Here's how the part is built. I have some questions about the finished solid (model axes, mm). Round coordinates to 2 decimals unless told otherwise and drop trailing zeros. Write each loop counter-clockwise with the first axis right and the second up, starting at its lowest first coordinate (ties: lowest second). Pieces come first, ordered by that corner, then holes. Notation, with made-up numbers: (70, 32) - (90, 32) arc R18 ccw to (90, 55) - close; hole circle Ø9 at (29.5, 26.25). An arc over 180 degrees is marked (long way). Use one line per item in the form item = value. Start each with the question number.
1. I want a section at A-A, the plane x = 0. List the corners of the cut face in (y, z) for me, plus the area to 3 significant figures.
2. I want a section at C-C, the plane z = -65. List the corners of the cut face in (x, y) for me.
3. If I drill on line 1 along Z through (x, y) = (0, 2.25); line 2 along X through (y, z) = (1.25, -93.5); line 3 along X through (y, z) = (0, -108), over which ranges is the centre line in solid material (lowest first)?
4. Will these pins go through, and if not, where does the flat tip stop? pin 1 (4 mm diameter, centred on y = 1.5, z = -37, fed in from +X); pin 2 (3 mm diameter, centred on y = -2, z = -0.5, fed in from +X); pin 3 (3 mm diameter, centred on x = -1.5, y = 2.5, fed in from +Z); pin 4 (1.5 mm diameter, centred on x = -1.5, z = -55.5, fed in from -Y).
Autodesk Inventor part; units mm, degrees
ref_plane "FDT_KSAUFSATZ_XY" through (0, 0, 8.2) normal (0, 0, 1) x (-1, 0, 0)
ref_plane "FDT_KSAUFSATZ_YZ" through (0, 0, 8.2) normal (-1, 0, 0) x (0, -1, 0)
ref_plane "FDT_KSAUFSATZ_ZX" through (0, 0, 8.2) normal (0, -1, 0) x (0, 0, 1)
sketch "Sketch_2" plane through (0, 0, 0) normal (1, 0, 0) x (0, 1, 0)
  line L0 (0, -133.5) -> (0, 4)
  line L1 (0, 4) -> (2, 4)
  line L2 (2, 4) -> (2, -131.5)
  line L3 (2, -131.5) -> (4, -131.5)
  line L4 (4, -131.5) -> (4, -133.5)
  line L5 (4, -133.5) -> (0, -133.5)
  line L6 (0, -133.5) -> (0, 4)
revolve "Revolution1" add sketch "Sketch_2" angle 360 about axis through (0, 0, -133.5) along (0, 0, -1)
sketch "Sketch_6" plane through (0, 0, 0) normal (1, 0, 0) x (0, 1, 0)
  line L0 (0, 3) -> (0, 16)
  line L1 (0, 16) -> (1.5705, 16)
  line L2 (1.5705, 16) -> (2, 15.5705)
  line L3 (2, 15.5705) -> (2, 6.299)
  line L4 (2, 6.299) -> (1.6241, 5.2663)
  arc A0 (1.6241, 5.2663) -> (1.6, 5.1295) centre (2, 5.1295) ccw
  line L5 (1.6, 5.1295) -> (1.6, 4.4)
  arc A1 (1.6, 4.4) -> (2, 4) centre (2, 4.4) ccw
  line L6 (2, 4) -> (2, 3)
  line L7 (2, 3) -> (0, 3)
  line L8 (0, 3) -> (0, 16)
revolve "Revolution2" add sketch "Sketch_6" angle 360 about axis through (0, 0, 3) along (0, 0, -1)
thread "Thread1"
ref_plane "FDT_KSAUFSATZ_XY" through (0, 0, 8.2) normal (0, 0, 1) x (-1, 0, 0)
ref_plane "FDT_KSAUFSATZ_YZ" through (0, 0, 8.2) normal (-1, 0, 0) x (0, -1, 0)
ref_plane "FDT_KSAUFSATZ_ZX" through (0, 0, 8.2) normal (0, -1, 0) x (0, 0, 1)
ref_plane "FDT_NUT_XY" through (0, 0, 8.2) normal (0, 0, 1) x (-1, 0, 0)
ref_plane "FDT_NUT_YZ" through (0, 0, 8.2) normal (-1, 0, 0) x (0, -1, 0)
ref_plane "FDT_NUT_ZX" through (0, 0, 8.2) normal (0, -1, 0) x (0, 0, 1)
ref_plane "KS_XY" through (0, 0, 0) normal (0, 0, -1) x (1, 0, 0)
ref_plane "KS_YZ" through (0, 0, 0) normal (1, 0, 0) x (0, -1, 0)
ref_plane "KS_ZX" through (0, 0, 0) normal (0, -1, 0) x (0, 0, -1)
ref_plane "NUT1_XY" through (0, 0, 12) normal (0, 0, 1) x (1, 0, 0)
ref_plane "NUT1_YZ" through (0, 0, 12) normal (1, 0, 0) x (0, 1, 0)
ref_plane "NUT1_ZX" through (0, 0, 12) normal (0, 1, 0) x (0, 0, 1)
properties part number "19182 DSNU-8-100-P---(A---00--0-KS)"
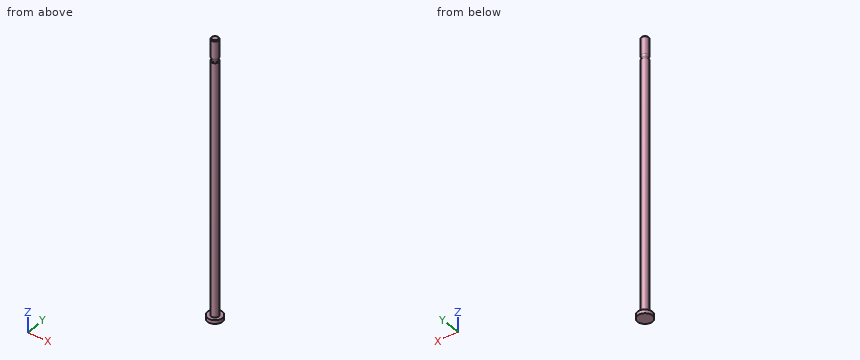
Model answer:
q1.outline = (-4, -133.5) - (4, -133.5) - (4, -131.5) - (2, -131.5) - (2, 4) arc R0.4 cw to (1.6, 4.4) - (1.6, 5.13) arc R0.4 cw to (1.62, 5.27) - (2, 6.3) - (2, 15.57) - (1.57, 16) - (-1.57, 16) - (-2, 15.57) - (-2, 6.3) - (-1.62, 5.27) arc R0.4 cw to (-1.6, 5.13) - (-1.6, 4.4) arc R0.4 cw to (-2, 4) - (-2, -131.5) - (-4, -131.5) - close
q1.area = 604 mm2
q2.outline = circle Ø4 at (0, 0)
q3.line_1 = -133.5 to -131.5
q3.line_2 = -1.56 to 1.56
q3.line_3 = -2 to 2
q4.pin_1 = 2
q4.pin_2 = 1.94
q4.pin_3 = 16
q4.pin_4 = -1.85
